```python
from build123d import *

# Parameters (mm, degrees)
SKIZZE1_R                            = 11
AUFSATZ_LINEAR_AUSTRAGEN1_DEPTH      = 30
SKIZZE2_R                            = 3
SCHNITT_LINEAR_AUSTRAGEN1_DEPTH      = 34.793490497
SKIZZE3_W                            = 30
SKIZZE3_H                            = 2
SCHNITT_LINEAR_AUSTRAGEN2_DEPTH      = 10
SCHNITT_LINEAR_AUSTRAGEN3_DEPTH      = 35.132096332
SCHNITT_LINEAR_AUSTRAGEN3_DEPTH_BACK = 35.132096332
SKIZZE4_R                            = 1
SKIZZE5_R                            = 1
SCHNITT_LINEAR_AUSTRAGEN4_DEPTH      = 10


with BuildPart() as part:
    # Skizze1 → Aufsatz-Linear austragen1 (new body)
    with BuildSketch(Plane(origin=(0, 0, 0), x_dir=(1, 0, 0), z_dir=(0, 1, 0))):
        with Locations(Location((0, 0, 0), (0, 0, 270))):
            Circle(SKIZZE1_R)
    extrude(amount=AUFSATZ_LINEAR_AUSTRAGEN1_DEPTH)

    # Skizze2 → Schnitt-Linear austragen1 (cut, through all)
    with BuildSketch(Plane(origin=(0, 30, 0), x_dir=(1, 0, 0), z_dir=(0, 1, 0))):
        with Locations(Location((0, 0, 0), (0, 0, 270))):
            Circle(SKIZZE2_R)
    extrude(amount=-SCHNITT_LINEAR_AUSTRAGEN1_DEPTH, mode=Mode.SUBTRACT)

    # Skizze3 → Schnitt-Linear austragen2 (cut)
    with BuildSketch(Plane(origin=(0, 30, 0), x_dir=(1, 0, 0), z_dir=(0, 1, 0))):
        Rectangle(SKIZZE3_W, SKIZZE3_H)
    extrude(amount=-SCHNITT_LINEAR_AUSTRAGEN2_DEPTH, mode=Mode.SUBTRACT)

    # Skizze4 → Schnitt-Linear austragen3 (cut, two sides: drawn at the far end of the back side and taken through both)
    with BuildSketch(Plane.XY.offset(-1).offset(-SCHNITT_LINEAR_AUSTRAGEN3_DEPTH_BACK)):
        with Locations((0, 26)):
            Circle(SKIZZE4_R)
    extrude(amount=SCHNITT_LINEAR_AUSTRAGEN3_DEPTH + SCHNITT_LINEAR_AUSTRAGEN3_DEPTH_BACK, mode=Mode.SUBTRACT)

    # Skizze5 → Schnitt-Linear austragen4 (cut)
    with BuildSketch(Plane.XZ):
        with Locations(Location((0, 7.5, 0), (0, 0, 270))):
            Circle(SKIZZE5_R)
        with Locations(Location((0, -7.5, 0), (0, 0, 270))):
            Circle(SKIZZE5_R)
    extrude(amount=-SCHNITT_LINEAR_AUSTRAGEN4_DEPTH, mode=Mode.SUBTRACT)


solid = part.part
```
Read the model definition and answer for the solid it produces. Units are mm, in the model's axes. A direction names the side the tool comes from. Give positions to 0.01 mm unless a question says otherwise; leave off trailing zeros. Write each loop counter-clockwise with the first axis right and the second up, starting at its lowest first coordinate (ties: lowest second). Pieces come first, ordered by that corner, then holes. Notation, with made-up numbers: (7, -19.75) -> (63, -19.75) arc R18 cw to (63, 13.25) -> close; hole circle Ø9 at (37.25, -8). An arc over 180 degrees is marked (long way). Answer as a JSON object with one key per item and string values.
1) Section A-A on z = 0 is taken. Write down the section's boundary in (x, y), then the cut area to 3 significant figures.
Findings below:
{"outline": "(-11, 0) -> (-3, 0) -> (-3, 20) -> (-11, 20) -> close; (3, 0) -> (11, 0) -> (11, 20) -> (3, 20) -> close", "area": "320 mm^2"}
2) Section C-C on x = 0 is taken. Write down the section's boundary in (y, z), then the cut area to 3 significant figures.
Findings below:
{"outline": "(0, -11) -> (25, -11) -> (25, -3) -> (0, -3) -> (0, -6.5) -> (10, -6.5) -> (10, -8.5) -> (0, -8.5) -> close; (0, 3) -> (25, 3) -> (25, 11) -> (0, 11) -> (0, 8.5) -> (10, 8.5) -> (10, 6.5) -> (0, 6.5) -> close; (27, -11) -> (30, -11) -> (30, -3) -> (27, -3) -> close; (27, 3) -> (30, 3) -> (30, 11) -> (27, 11) -> close", "area": "408 mm^2"}
3) Straight lines are drawn through the part: probe 1 along Y at (x, z) = (0, 5.5); probe 2 along Y at (x, z) = (0, -7); probe 3 along X at (y, z) = (12.5, 0). For each, find the intervals that lie inside material, in ascending order. Write a range as from..to.
Findings below:
{"probe 1": "y = 0..25, 27..30", "probe 2": "y = 10..25, 27..30", "probe 3": "x = -11..-3, 3..11"}
4) Section D-D on z = 7.5 is taken. Write down the section's boundary in (x, y).
Findings below:
{"outline": "(-8.05, 0) -> (-1, 0) -> (-1, 10) -> (1, 10) -> (1, 0) -> (8.05, 0) -> (8.05, 30) -> (-8.05, 30) -> close; hole circle Ø2 at (0, 26)"}
5) A tool of negligible diameter and unlimited length cuts with its end or side. For faces 1 (the cylindrical face through (0, 25, 7)), 2 (the flat face through (7, 20, 0)), 3 (the cylindrical face through (-0.6, 4.9, 8.3)), from which of +Z, -Z, +X, -X, +Y, -Y can it reach the whole face along a straight path? Write none if from no direction.
Findings below:
{"face 1": "+Z, -Z", "face 2": "+X, -X, +Y", "face 3": "-Y"}
6) For a pull along X with two mould halves and no side action, classify faces 4 (the cylindrical face through (-0.6, 4.9, -6.7)), 5 (the flat face through (7, 25, 1)), 6 (the cylindrical face through (-10.74, 14.79, -2.38)) as pulls with the +X half, pulls with the -X half, needs draft (parallel to the pull), parting line crosses it, or undercut.
Findings below:
{"face 4": "undercut", "face 5": "needs draft", "face 6": "parting line crosses it"}
7) Flat-ended cylindrical pins translate along their axes: pin 1 Ø10 at (x, y) = (5.5, 25) entering from -Z; pin 2 Ø4 at (x, y) = (5, 25) entering from +Z; pin 3 Ø4 at (x, y) = (-8, 26) entering from -Z; pin 4 Ø5.5 at (x, z) = (0, 0) entering from +Y. Find the tip coordinate at first contact, or state that the pin passes through.
Findings below:
{"pin 1": "stops at z = -10.99", "pin 2": "stops at z = 10.58", "pin 3": "stops at z = -9.22", "pin 4": "passes through"}
